For this review, use the dimensioned drawing (mm, ordinates from the lowest corner) and the shaded views. A direction names the side the tool comes from. Coordinates: 2 decimals unless noted, no trailing zeros. Write each loop counter-clockwise with the first axis right and the second up, starting at its lowest first coordinate (ties: lowest second). Pieces come first, ordered by that corner, then holes. Notation, with made-up numbers: M -10.75,87.5 L 27.25,87.5 A14 ccw 27.25,109.5 Z; hole C 64.5,54 d7. An arc over 180 degrees is marked long. One line per question, with ' | ' between items.
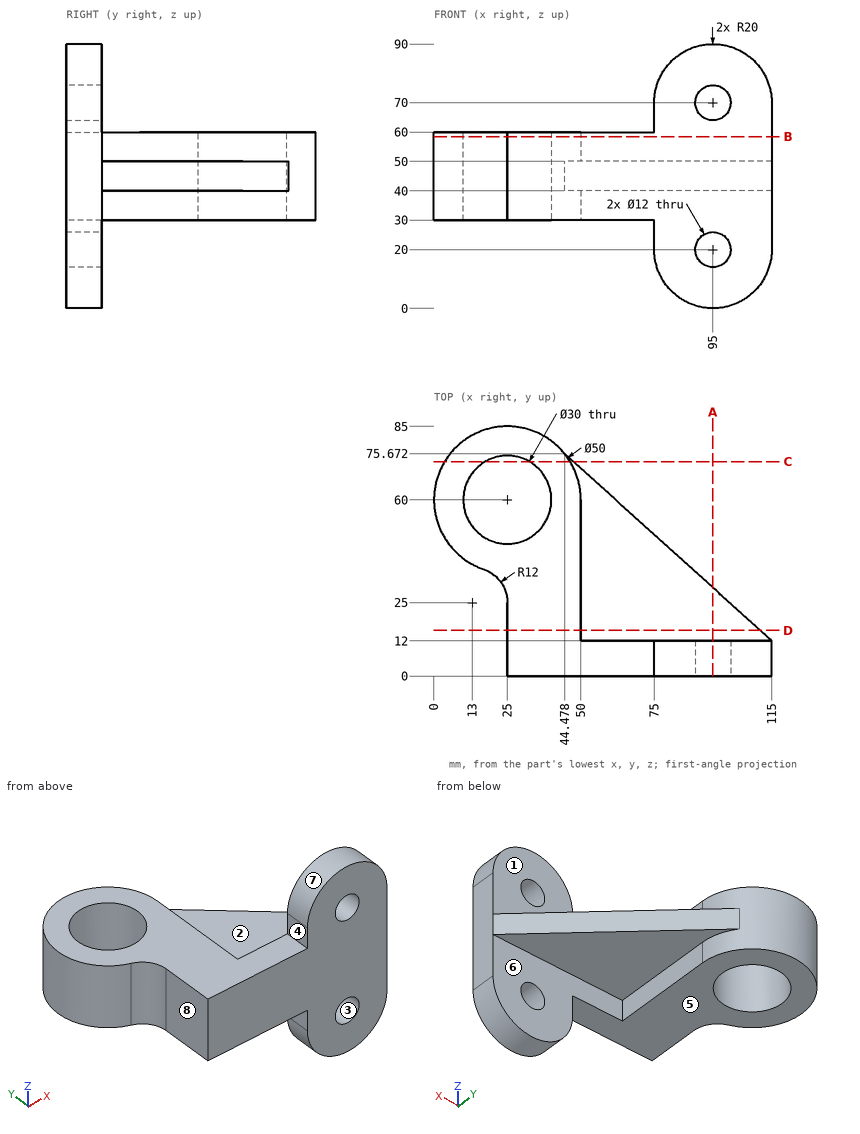
1. To check wall thickness, follow line 1 along X through (y, z) = (2.5, 20); line 2 along Z through (x, y) = (33, 77); line 3 along Y through (x, z) = (94, 76). State the ranges of each line that lie inside material, in increasing order. Write a range as [from, to].
Answer sheet:
line 1: [75, 89], [101, 115] | line 2: [30, 60] | line 3: [0, 12]
2. Take a section at D-D (y = 15.5). Write out the cut boundary in (x, z), then the cut area to 3 significant figures.
Answer sheet:
outline: M 25,30 L 50,30 L 50,40 L 111.12,40 L 111.12,50 L 50,50 L 50,60 L 25,60 Z | area: 1,360 mm^2
3. Insertion check: pin 1 Ø5 at (y, z) = (4.5, 64.5) entering from -X; pin 2 Ø20 at (x, z) = (92, 68) entering from +Y; pin 3 Ø12 at (x, y) = (44.5, 58) entering from -Z; pin 4 Ø4 at (y, z) = (13.5, 39.5) entering from +X. Each pin has a flat end and moves straight along its axis. Give the tip position at first contact, or say it passes through.
Answer sheet:
pin 1: x = 75 | pin 2: y = 12 | pin 3: z = 30 | pin 4: x = 115
4. Draft analysis for pull direction Z (two halves, no side actions). For the marked faces 1, 2 and 3, state which applies: pulls with the +Z half, pulls with the -Z half, needs draft (parallel to the pull), parting line crosses it, or undercut.
Answer sheet:
face 1: needs draft | face 2: pulls with the +Z half | face 3: undercut
5. Tool access review of the marked faces 4, 5, 6, 7 and 8: name each direction out of +Z, -Z, +X, -X, +Y, -Y from which nothing blocks a thin tool from reaching the whole face with its end or side.
Answer sheet:
face 4: +Z, -X, +Y, -Y | face 5: -Z, -X, +Y, -Y | face 6: -Z, +X, +Y | face 7: +Z, +Y, -Y | face 8: +Z, -Z, -X, -Y
6. Take a section at A-A (x = 95). Write out the cut boundary in (y, z).
Answer sheet:
outline: M 0,0 L 12,0 L 12,14 L 0,14 Z; M 0,26 L 12,26 L 12,40 L 30.06,40 L 30.06,50 L 12,50 L 12,64 L 0,64 Z; M 0,76 L 12,76 L 12,90 L 0,90 Z
7. Take a section at C-C (y = 73). Write out the cut boundary in (x, z), then the cut area to 3 significant figures.
Answer sheet:
outline: M 3.65,30 L 17.52,30 L 17.52,60 L 3.65,60 Z; M 32.48,30 L 46.35,30 L 46.35,40 L 47.44,40 L 47.44,50 L 46.35,50 L 46.35,60 L 32.48,60 Z | area: 843 mm^2
8. Take a section at B-B (z = 58.5). Write out the cut boundary in (x, y), then the cut area to 3 significant figures.
Answer sheet:
outline: M 16.89,36.35 A12 cw 25,25 L 25,0 L 115,0 L 115,12 L 50,12 L 50,60 A25 ccw long Z; hole C 25,60 d30 | area: 3,060 mm^2
